The listing builds one solid part. Answer for the finished solid, in the listing's coordinates (mm). A direction names the side the tool comes from. Round coordinates to 2 decimals unless told otherwise and drop trailing zeros. Loops run counter-clockwise (first coordinate to the right, second up) from the corner with the lowest first, then second, coordinate; pieces in that order, holes last. Notation, with made-up numbers: (-12.75, -38.5) -> (0.25, -38.5) arc R11 ccw to (0.25, -28.5) -> close; hole circle Ø10 at (14.25, 57.5). An arc over 180 degrees is marked (long way). Use a Markdown table: item, result. Add a question column.
Q1. Given pin 1 Ø1 at (x, z) = (3.5, 26) entering from +Y; pin 2 Ø2.5 at (x, y) = (-31.75, 0) entering from +Z, each flat-ended and moving along its own axis, determine where each tip first touches the part or whether it passes through.
Q2. Section A-A on x = -31.75 is taken. Give the vertices of the cut face in (y, z) (1 decimal), then the cut area to 3 significant figures.
Q3. Which of the six approach directions +Z, -Z, +X, -X, +Y, -Y give full straight-line access (tool end or side, diameter ignored) to faces 1 (the flat face through (-33, 1, 3)), 2 (the cylindrical face through (30.734, -0.421, 1.479)), 3 (the flat face through (-25.4, 0, 2)), 4 (the flat face through (33, 1, 3))?
Q4. Section B-B on y = 0 is taken. Give the number of separate pieces and of enclosed holes in the cut face, then the cut area to 3 significant figures.
Q5. Consider line 1 (X direction, y = -1, z = 10.5); line 2 (X direction, y = 0.75, z = 22); line 3 (X direction, y = 0.75, z = 1) (3 decimals). Determine where each line is inside the solid, lowest interval first.
Q6. For a pull along X with two mould halves and no side action, classify faces 5 (the cylindrical face through (-30.734, -0.421, 1.479)), 6 (the flat face through (-34.925, 0, 1)), 7 (the flat face through (-30, 0, 0)) as released by +X, released by -X, zero draft, split by the parting line, or undercut.
from build123d import *

# Parameters (mm, degrees)
SKETCH2_W           = 6.35
SKETCH2_H           = 6.35
SKETCH2_R           = 1.1
BOSS_EXTRUDE1_DEPTH = 3
SKETCH4_W           = 3.175
SKETCH4_H           = 6.35
FILLET1_R           = 1
FILLET3_R           = 0.79375


with BuildPart() as part:
    # Sketch2 → Boss-Extrude1 (new body)
    with BuildSketch(Plane.XY):
        with Locations((-31.75, 0)):
            Rectangle(SKETCH2_W, SKETCH2_H)
        with Locations((-31.75, 0)):
            Circle(SKETCH2_R, mode=Mode.SUBTRACT)
    extrude(amount=BOSS_EXTRUDE1_DEPTH)

    # Sweep1: sweep along a path in Sketch3
    with BuildLine(Plane(origin=(0, 0, 0), x_dir=(1, 0, 0), z_dir=(0, 1, 0))) as sweep1_path:
        Line((-28.575, 0), (-28.575, -3))
        ThreePointArc((-28.575, -3), (-20.205576272, -23.205576272), (0, -31.575))
    # Sketch4 → Sweep1 (sweep)
    with BuildSketch(Plane.XY):
        with Locations((-26.9875, 0)):
            Rectangle(SKETCH4_W, SKETCH4_H)
    sweep(path=sweep1_path.line)

    # Fillet1
    fillet1_edges = [part.edges().sort_by_distance(p)[0] for p in [
        (-28.575, 0, 3),
    ]]
    fillet(fillet1_edges, radius=FILLET1_R)

    # Fillet3
    fillet3_edges = [part.edges().sort_by_distance(p)[0] for p in [
        (-25.4, 3.175, 1.5),
        (-25.4, -3.175, 1.5),
        (-17.960512242, 3.175, 20.960512242),
        (-17.960512242, -3.175, 20.960512242),
        (-19.861039911, -3.175, 23.54433544),
        (-28.863039479, -3.175, 3.28103813),
        (-19.861039911, 3.175, 23.54433544),
        (-28.863039479, 3.175, 3.28103813),
        (-32.241544497, -3.175, 3),
        (-34.925, 0, 3),
        (-34.925, 3.175, 1.5),
        (-34.925, -3.175, 1.5),
        (-32.241544497, 3.175, 3),
    ]]
    fillet(fillet3_edges, radius=FILLET3_R)

    # Mirror1: part across plane


with BuildPart() as part_1:
    add(part.part)
    add(part.part.mirror(Plane(origin=(0, 0, 3), x_dir=(0, 0, 1), z_dir=(1, 0, 0))))


solid = part_1.part
Checked values:
| question | item | result |
|---|---|---|
| 1 | pin 1 | passes through |
| 1 | pin 2 | stops at z = 3 |
| 2 | outline | (-3.2, 0) -> (-1.1, 0) -> (-1.1, 3) -> (-2.4, 3) arc R0.8 ccw to (-3.2, 2.2) -> close; (1.1, 0) -> (3.2, 0) -> (3.2, 2.2) arc R0.8 ccw to (2.4, 3) -> (1.1, 3) -> close |
| 2 | area | 12.2 mm2 |
| 3 | face 1 | +Z, -X, +Y, -Y |
| 3 | face 2 | +Z, -Z |
| 3 | face 3 | -Z, +Y, -Y |
| 3 | face 4 | +Z, +X, +Y, -Y |
| 4 | separate pieces | 3 |
| 4 | enclosed holes | 0 |
| 4 | area | 313 mm2 |
| 5 | line 1 | x = -27.57 to -24.27, 24.27 to 27.57 |
| 5 | line 2 | x = -21.34 to -16.86, 16.86 to 21.34 |
| 5 | line 3 | x = -34.925 to -32.555, -30.945 to -25.4, 25.4 to 30.945, 32.555 to 34.925 |
| 6 | face 5 | undercut |
| 6 | face 6 | released by -X |
| 6 | face 7 | zero draft |
